Read the model definition and answer for the solid it produces. Units are mm, in the model's axes. Face numbers are marked on the shaded views. A direction names the side the tool comes from. Give positions to 0.01 mm unless a question says otherwise; leave off trailing zeros. Write each loop counter-clockwise with the first axis right and the second up, starting at its lowest first coordinate (ties: lowest second). Pieces come first, ordered by that corner, then holes. Notation, with made-up numbers: M -26,56 L 0,56 A25 cw 0,81 Z; hole C 79.5,-12 d5. An arc over 180 degrees is marked long. Answer as CSV lines item,"result". Start each with the question number.
```python
from build123d import *

# Parameters (mm, degrees)
SKETCH1_R           = 1.875
BOSS_EXTRUDE1_DEPTH = 1.2
SKETCH2_R           = 1
BOSS_EXTRUDE2_DEPTH = 12


with BuildPart() as part:
    # Sketch1 → Boss-Extrude1 (new body)
    with BuildSketch(Plane(origin=(0, 0, 0), x_dir=(1, 0, 0), z_dir=(0, 1, 0))):
        with Locations(Location((0, 0, 0), (0, 0, 270))):
            Circle(SKETCH1_R)
        Polygon((0.866025404, 0), (0.433012702, 0.75), (-0.433012702, 0.75), (-0.866025404, 0), (-0.433012702, -0.75), (0.433012702, -0.75), align=None, mode=Mode.SUBTRACT)
    extrude(amount=BOSS_EXTRUDE1_DEPTH)

    # Sketch2 → Boss-Extrude2 (add)
    with BuildSketch(Plane(origin=(0, 1.2, 0), x_dir=(1, 0, 0), z_dir=(0, 1, 0))):
        with Locations(Location((0, 0, 0), (0, 0, 270))):
            Circle(SKETCH2_R)
    extrude(amount=BOSS_EXTRUDE2_DEPTH)


solid = part.part
```
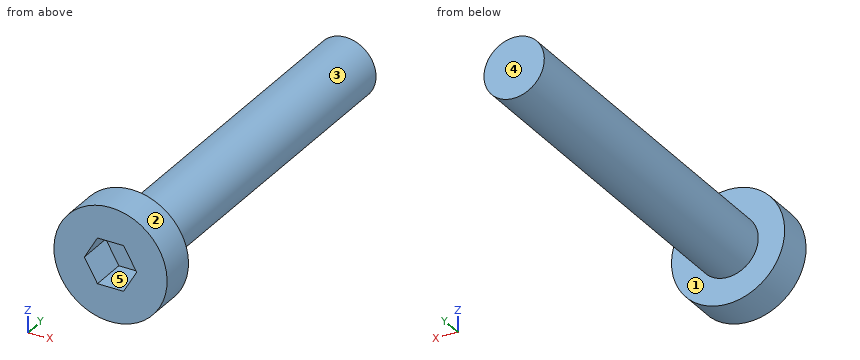
1. Find section A-A on x = 0. Determine the outline of the cut face in (y, z) (3 decimals), then the cut area to 3 significant figures.
2. Given pin 1 (1.2 mm diameter, centred on x = 0, z = 0, fed in from -Y); pin 2 (1.5 mm diameter, centred on x = 1.5, z = -1, fed in from +Y), each flat-ended and moving along its own axis, determine where each tip first touches the part or whether it passes through.
3. For the marked faces 1 and 2, determine the directions among +Z, -Z, +X, -X, +Y, -Y from which every point of the face is accessible in a straight line to the end or side of a thin tool.
4. Find the intervals of material crossed by line 1 (Y direction, x = -1.45, z = 0.05); line 2 (Y direction, x = -0.2, z = -0.45); line 3 (X direction, y = 4, z = 0), in increasing order. Write a range as [from, to].
5. Find section D-D on x = 1.65. Determine the outline of the cut face in (y, z).
6. Find section B-B on z = -0.4. Determine the outline of the cut face in (x, y).
7. Find section C-C on y = 7.5. Determine the outline of the cut face in (x, z), then the cut area to 3 significant figures.
8. Determine the mould class of the marked faces 3, 4 and 5 for opening direction Z: +Z half, -Z half, draft (parallel to the pull), parting line (faces both ways), or undercut.
Computed:
1,outline,"M 0,-1.875 L 1.2,-1.875 L 1.2,-1 L 13.2,-1 L 13.2,1 L 1.2,1 L 1.2,1.875 L 0,1.875 L 0,0.75 L 1.2,0.75 L 1.2,-0.75 L 0,-0.75 Z"
1,area,"26.7 mm^2"
2,pin 1,"stops at y = 1.2"
2,pin 2,"stops at y = 1.2"
3,face 1,"+Y"
3,face 2,"+Y, -Y"
4,line 1,"y = [0, 1.2]"
4,line 2,"y = [1.2, 13.2]"
4,line 3,"x = [-1, 1]"
5,outline,"M 0,-0.89 L 1.2,-0.89 L 1.2,0.89 L 0,0.89 Z"
6,outline,"M -1.83,0 L -0.64,0 L -0.64,1.2 L 0.64,1.2 L 0.64,0 L 1.83,0 L 1.83,1.2 L 0.92,1.2 L 0.92,13.2 L -0.92,13.2 L -0.92,1.2 L -1.83,1.2 Z"
7,outline,"C 0,0 d2"
7,area,"3.14 mm^2"
8,face 3,"parting line"
8,face 4,"draft"
8,face 5,"undercut"
